```python
from build123d import *

# Parameters (mm, degrees)
F0_R     = 3.25
F1_DEPTH = 10


with BuildPart() as f1:
    # F0 (on Front) → F1 (new body)
    with BuildSketch(Plane.XZ):
        with BuildLine():
            Line((-13.4, -9.5), (-13.4, -6.540226))
            Line((-13.4, -6.540226), (-15.4, -6.540226))
            Line((-15.4, -6.540226), (-15.4, -11.55))
            Line((-15.4, -11.55), (15.4, -11.55))
            Line((15.4, -11.55), (15.4, -6.540226))
            Line((15.4, -6.540226), (13.4, -6.540226))
            Line((13.4, -6.540226), (13.4, -9.5))
            Line((13.4, -9.5), (13.4, -9.55))
            Line((13.4, -9.55), (12.2, -9.55))
            Line((12.2, -9.55), (12.2, -9.5))
            Line((12.2, -9.5), (12.2, 5.5))
            ThreePointArc((12.2, 5.5), (11.32132, 7.62132), (9.2, 8.5))
            Line((9.2, 8.5), (-9.2, 8.5))
            ThreePointArc((-9.2, 8.5), (-11.32132, 7.62132), (-12.2, 5.5))
            Line((-12.2, 5.5), (-12.2, -9.5))
            Line((-12.2, -9.5), (-12.2, -9.55))
            Line((-12.2, -9.55), (-13.4, -9.55))
            Line((-13.4, -9.55), (-13.4, -9.5))
        make_face()
        with Locations((0, -1.5)):
            Circle(F0_R, mode=Mode.SUBTRACT)
    extrude(amount=F1_DEPTH)


solid = f1.part
```
Verification items for the finished model (mm, model axes). A direction names the side the tool comes from. Give positions to 0.01 mm unless a question says otherwise; leave off trailing zeros. Write each loop counter-clockwise with the first axis right and the second up, starting at its lowest first coordinate (ties: lowest second). Pieces come first, ordered by that corner, then holes. Notation, with made-up numbers: M 73,86 L 90,86 A34 cw 90,122 Z; hole C 70,-16.75 d2. An arc over 180 degrees is marked long. One line per question, with ' | ' between items.
1) Gauge pin test, flat ends, axial feed: pin 1 Ø5 at (y, z) = (-6, -3.5) entering from +X; pin 2 Ø1.6 at (x, y) = (15, -3) entering from +Z; pin 3 Ø0.6 at (x, y) = (13, -3) entering from +Z. Record the tip position at first contact, or that the pin passes through.
Result:
pin 1: stops at x = 12.2 | pin 2: stops at z = -6.54 | pin 3: stops at z = -9.55
2) Section check C-C on y = -4.5. Enter the section's corners in (x, z).
Result:
outline: M -15.4,-11.55 L 15.4,-11.55 L 15.4,-6.54 L 13.4,-6.54 L 13.4,-9.55 L 12.2,-9.55 L 12.2,5.5 A3 ccw 9.2,8.5 L -9.2,8.5 A3 ccw -12.2,5.5 L -12.2,-9.55 L -13.4,-9.55 L -13.4,-6.54 L -15.4,-6.54 Z; hole C 0,-1.5 d6.5
3) Section check D-D on z = 3.75. Enter the section's corners in (x, y).
Result:
outline: M -12.2,-10 L 12.2,-10 L 12.2,0 L -12.2,0 Z
4) Section check A-A on z = -1.5. Enter the section's corners in (x, y), plus the area to 3 significant figures.
Result:
outline: M -12.2,-10 L -3.25,-10 L -3.25,0 L -12.2,0 Z; M 3.25,-10 L 12.2,-10 L 12.2,0 L 3.25,0 Z | area: 179 mm2
5) Mould release check, pull along X, two halves, no side actions. Record for faces 1 (the flat face through (13.4, -5, -8)), 2 (the flat face through (-4, -10, -1)), 3 (the flat face through (15.4, -5, -9)), 4 (the flat face through (-13.4, -5, -8)): released by +X, released by -X, zero draft, split by the parting line, or undercut.
Result:
face 1: undercut | face 2: zero draft | face 3: released by +X | face 4: undercut
6) Thickness scan on line 1 along X through (y, z) = (-6, -8.75); line 2 along Z through (x, y) = (0, -6); line 3 along Z through (x, y) = (-12.5, -9). Record the ranges inside material, lowest first. Write a range as [from, to].
Result:
line 1: x = [-15.4, -13.4], [-12.2, 12.2], [13.4, 15.4] | line 2: z = [-11.55, -4.75], [1.75, 8.5] | line 3: z = [-11.55, -9.55]
7) Set-up check for faces 5 (the flat face through (13, -5, -9.55)), 6 (the flat face through (-14, -5, -6.54)), 7 (the cylindrical face through (-2.579, -4.93, -3.478)), 8 (the flat face through (0, -5, 8.5)), 9 (the flat face through (14, -5, -6.54)): record each of +Z, -Z, +X, -X, +Y, -Y from which the full face is reachable in a straight line by a thin tool's end or side.
Result:
face 5: +Z, +Y, -Y | face 6: +Z, -X, +Y, -Y | face 7: +Y, -Y | face 8: +Z, +X, -X, +Y, -Y | face 9: +Z, +X, +Y, -Y
8) Section check B-B on x = 0. Enter the section's corners in (y, z), plus the area to 4 significant figures.
Result:
outline: M -10,-11.55 L 0,-11.55 L 0,-4.75 L -10,-4.75 Z; M -10,1.75 L 0,1.75 L 0,8.5 L -10,8.5 Z | area: 135.5 mm2
